from build123d import *

# Parameters (mm, degrees)
BOSS_EXTRUDE1_DEPTH = 15
SKETCH2_R           = 2.75
CUT_EXTRUDE1_DEPTH  = 19.05
SKETCH3_R           = 2.75
CUT_EXTRUDE2_DEPTH  = 26.416530054


with BuildPart() as part:
    # Sketch1 → Boss-Extrude1 (new body)
    with BuildSketch(Plane.XY):
        Polygon((0, 0), (0, 15), (1, 15), (1, 1), (15, 1), (15, 0), align=None)
    extrude(amount=BOSS_EXTRUDE1_DEPTH)

    # Sketch2 → Cut-Extrude1 (cut)
    with BuildSketch(Plane(origin=(0, 0, 0), x_dir=(-1, 0, 0), z_dir=(0, -1, 0))):
        with Locations(Location((-8, -7.5, 0), (0, 0, 180))):
            Circle(SKETCH2_R)
    extrude(amount=-CUT_EXTRUDE1_DEPTH, mode=Mode.SUBTRACT)

    # Sketch3 → Cut-Extrude2 (cut, through all)
    with BuildSketch(Plane(origin=(1, 0, 0), x_dir=(0, 0, -1), z_dir=(1, 0, 0))):
        with Locations(Location((-7.5, 8, 0), (0, 0, 90))):
            Circle(SKETCH3_R)
    extrude(amount=-CUT_EXTRUDE2_DEPTH, mode=Mode.SUBTRACT)


solid = part.part
Can you work these out from the model? Positions are in its coordinate system, mm. A direction names the side the tool comes from. Give positions to 0.01 mm unless a question says otherwise; leave off trailing zeros. Order: outer loops, then holes, each group sorted by start corner. A loop starts at its lowest first (then second) coordinate and runs counter-clockwise, first axis right, second up. Notation, with made-up numbers: M 81,-22.75 L 118,-22.75 A22 ccw 118,-8.75 Z; hole C 59,-34.75 d4. An arc over 180 degrees is marked long. Use a Markdown table: item, result. Add a question column.
Item 1: Suppose I cut it at A-A (y = 8). List the corners of the cut face in (x, z) for me.
Item 2: We'd pull the mould along Z, two halves only. Please class faces 1 (the flat face through (1, 11, 7)), 2 (the cylindrical face through (10.62, 0.49, 8.33)): +Z half, -Z half, draft (parallel to the pull), parting line (faces both ways), or undercut.
Item 3: Will these pins go through, and if not, where does the flat tip stop? pin 1 (3 mm diameter, centred on y = 11.5, z = 2.5, fed in from +X); pin 2 (6.5 mm diameter, centred on x = 8, z = 7.5, fed in from +Y).
Item 4: Suppose I cut it at D-D (z = 1). List the corners of the cut face in (x, y) for me, then the cut area to 3 significant figures.
Item 5: If I drill on L1, parallel to Z at x = 0.7, y = 8; L2, parallel to X at y = 12.5, z = 7.25, over which ranges is the centre line in solid material (lowest first)? Write a range as [from, to].
Item 6: For faces 3 (the flat face through (11, 1, 7)), 4 (the cylindrical face through (0.51, 10.62, 8.33)), which set-ups out of +Z, -Z, +X, -X, +Y, -Y let a thin tool reach every point of the face, with its end or its side?
Item 7: Suppose I cut it at B-B (z = 7.5). List the corners of the cut face in (x, y) for me, then the cut area to 3 significant figures.
Answer sheet:
| question | item | result |
|---|---|---|
| 1 | outline | M 0,0 L 1,0 L 1,4.75 L 0,4.75 Z; M 0,10.25 L 1,10.25 L 1,15 L 0,15 Z |
| 2 | face 1 | draft |
| 2 | face 2 | undercut |
| 3 | pin 1 | stops at x = 1 |
| 3 | pin 2 | stops at y = 1 |
| 4 | outline | M 0,0 L 15,0 L 15,1 L 1,1 L 1,15 L 0,15 Z |
| 4 | area | 29.0 mm² |
| 5 | L1 | z = [0, 4.75], [10.25, 15] |
| 5 | L2 | x = [0, 1] |
| 6 | face 3 | +Z, -Z, +X, +Y |
| 6 | face 4 | +X, -X |
| 7 | outline | M 0,0 L 5.25,0 L 5.25,1 L 1,1 L 1,5.25 L 0,5.25 Z; M 0,10.75 L 1,10.75 L 1,15 L 0,15 Z; M 10.75,0 L 15,0 L 15,1 L 10.75,1 Z |
| 7 | area | 18.0 mm² |
